Here's how the part is built. I have some questions about the finished solid (model axes, mm). Face numbers are marked on the shaded views. Give positions to 0.01 mm unless a question says otherwise; leave off trailing zeros. Write each loop counter-clockwise with the first axis right and the second up, starting at its lowest first coordinate (ties: lowest second). Pieces come first, ordered by that corner, then holes. Notation, with made-up numbers: M 85,45 L 102,45 A27 cw 102,73 Z; hole C -29,25.5 d3. An arc over 180 degrees is marked long. Answer as CSV lines item,"result". Start each with the question number.
Q1. Thinking about a two-plate mould opening in Y: for the marked faces 1, 2 and 3, which applies, +Y half, -Y half, draft (parallel to the pull), parting line (faces both ways), or undercut?
Q2. For pin 1 (12 mm diameter, centred on x = 87.5, y = 167, fed in from +Z); pin 2 (5 mm diameter, centred on x = -7.5, y = 89, fed in from -Z); pin 3 (5 mm diameter, centred on x = 17.5, y = 51.5, fed in from -Z); pin 4 (1.5 mm diameter, centred on x = 76.5, z = 27, fed in from +Y), each with a flat end and sliding along its axis, tell me the tip position at first contact or that it passes through.
Q3. Suppose I cut it at A-A (z = 0). Write out the boundary of the cut face in (x, y).
Q4. Suppose I cut it at B-B (x = 0). Write out the boundary of the cut face in (y, z).
Q5. Suppose I cut it at C-C (y = 101.6). Write out the boundary of the cut face in (x, z).
Q6. If I drill on line 1 along Z through (x, y) = (0, 74.5); line 2 along Z through (x, y) = (93.5, 101.6); line 3 along Y through (x, z) = (92, 0), over which ranges is the centre line in solid material (lowest first)?
Q7. Suppose I cut it at D-D (x = 72). Write out the boundary of the cut face in (y, z), then the cut area to 3 significant figures.
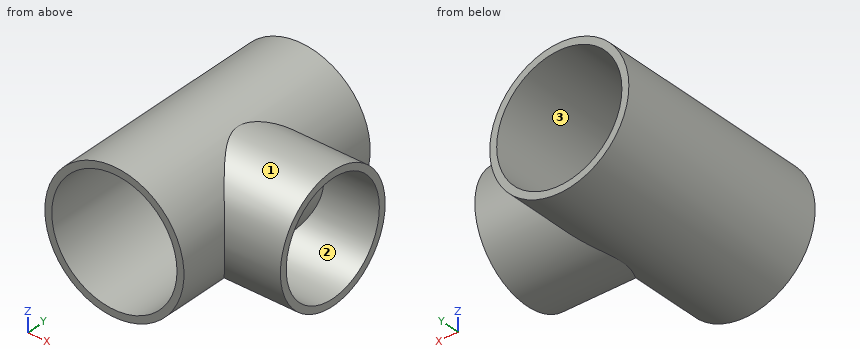
Autodesk Inventor part; units mm, degrees
ref_plane "Work Plane1" through (63.5, 0, 0) normal (1, 0, 0) x (0, 1, 0)
ref_plane "XZ Plane" through (0, 0, 0) normal (0, 1, 0) x (-1, 0, 0)
ref_plane "XY Plane" through (0, 0, 0) normal (0, 0, 1) x (1, 0, 0)
sketch "Sketch1" plane through (0, 0, 0) normal (0, 1, 0) x (-1, 0, 0)
  circle A0 centre (0, 0) radius 57.15
  circle A1 centre (0, 0) radius 63.5
  dimension "d0" = 114.3
  dimension "d1" = 6.35
extrude "Extrusion1" add sketch "Sketch1" along normal blind 203.2
ref_plane "Work Plane1" through (63.5, 0, 0) normal (1, 0, 0) x (0, 1, 0)
sketch "Sketch2" plane through (63.5, 0, 0) normal (1, 0, 0) x (0, 1, 0)
  circle A0 centre (101.6, 0) radius 57.15
  circle A1 centre (101.6, 0) radius 50.8
  point P0 (0, 0)
  dimension "d4" = 101.6
  dimension "d5" = 114.3
  dimension "d6" = 101.6
extrude "Extrusion2" add sketch "Sketch2" along normal blind 50.8 and the other way blind 63.5
sketch "Sketch3" plane through (0, 203.2, 0) normal (0, 1, 0) x (1, 0, 0)
  circle A0 centre (0, 0) radius 57.15
extrude "Extrusion3" cut sketch "Sketch3" against normal blind 254
properties part number "T Junction"
Resolved:
1,face 1,"parting line"
1,face 2,"undercut"
1,face 3,"draft"
2,pin 1,"through"
2,pin 2,"z = -63.3"
2,pin 3,"z = -61.7"
2,pin 4,"y = 152.36"
3,outline,"M -63.5,0 L -57.15,0 L -57.15,203.2 L -63.5,203.2 Z; M 57.15,0 L 63.5,0 L 63.5,44.45 L 114.3,44.45 L 114.3,50.8 L 63.5,50.8 L 63.5,152.4 L 114.3,152.4 L 114.3,158.75 L 63.5,158.75 L 63.5,203.2 L 57.15,203.2 Z"
4,outline,"M 0,-63.5 L 203.2,-63.5 L 203.2,-57.15 L 0,-57.15 Z; M 0,57.15 L 203.2,57.15 L 203.2,63.5 L 0,63.5 Z"
5,outline,"M 27.68,-57.15 L 114.3,-57.15 L 114.3,-50.8 L 38.1,-50.8 A63.5 ccw 38.1,50.8 L 114.3,50.8 L 114.3,57.15 L 27.68,57.15 A63.5 ccw long Z; hole C 0,0 d114.3"
6,line 1,"-63.5 to -57.15, 57.15 to 63.5"
6,line 2,"-57.15 to -50.8, 50.8 to 57.15"
6,line 3,"44.45 to 50.8, 152.4 to 158.75"
7,outline,"C 101.6,0 d114.3; hole C 101.6,0 d101.6"
7,area,"2,150 mm^2"
